The listing builds one solid part. Answer for the finished solid, in the listing's coordinates (mm). A direction names the side the tool comes from. Round coordinates to 2 decimals unless told otherwise and drop trailing zeros. Order: outer loops, then holes, each group sorted by start corner. A loop starts at its lowest first (then second) coordinate and runs counter-clockwise, first axis right, second up. Notation, with made-up numbers: (-2, -13) -> (51, -13) arc R22 ccw to (51, 25) -> close; hole circle Ø10 at (-4.5, -34.75). An arc over 180 degrees is marked (long way). Return JSON: item names as keys, results as strings. Group by question number.
(1) Which of the six approach directions +Z, -Z, +X, -X, +Y, -Y give full straight-line access (tool end or side, diameter ignored) to faces 5 (the face through (1589.699, -64, 595)), 6 (the face through (2161.199, -69, 594))?
(2) The part is cut by section A-A (z = 535.5). Determine the outline of the cut face in (x, y) (3 decimals), plus the area to 3 significant figures.
(3) The part is cut by section D-D (x = 1942.5). Determine the outline of the cut face in (y, z) (3 decimals), plus the area to 3 significant figures.
(4) Consider line 1 (Z direction, x = 1769, y = -71.5); line 2 (X direction, y = -91, z = 638); line 3 (Y direction, x = 1676.5, z = 332) (3 decimals). Determine where each line is inside the solid, lowest interval first. Write a range as [from, to].
(5) The part is cut by section C-C (y = -76.5). Determine the outline of the cut face in (x, z).
(6) Determine the mould class of faces 1 (the face through (1840.956, 4.696, 556.211)), 2 (the face through (1899, -64, 895.149)), 3 (the face through (1890, -64, 285.549)), 4 (the face through (1898, -69, 323.649)) for opening direction Z: +Z half, -Z half, draft (parallel to the pull), parting line (faces both ways), or undercut.
(7) The part is cut by section B-B (x = 1684). Determine the outline of the cut face in (y, z) (3 decimals), plus the area to 3 significant figures.
(8) This flat-tipped pin is pushed along its axis until it touches: pin 1 (2 mm diameter, centred on x = 1862, z = 490.5, fed in from -Y). Where does it stop, or does it pass through?
from build123d import *

# Parameters (mm, degrees)
SKETCH1_W           = 609.6
SKETCH1_H           = 609.6
SKETCH1_R           = 63.5
BOSS_EXTRUDE1_DEPTH = 9.525
BOSS_EXTRUDE2_DEPTH = 139.7


with BuildPart() as part:
    # Sketch1 → Boss-Extrude1 (new body)
    with BuildSketch(Plane(origin=(0, 0, 0), x_dir=(1, 0, 0), z_dir=(0, 1, 0))):
        with Locations((1894.49897269, -590.348674534)):
            Rectangle(SKETCH1_W, SKETCH1_H)
        with Locations(Location((1894.49897269, -590.348674534, 0), (0, 0, 90))):
            Circle(SKETCH1_R, mode=Mode.SUBTRACT)
    extrude(amount=BOSS_EXTRUDE1_DEPTH)

    # Sketch2 → Boss-Extrude2 (add)
    with BuildSketch(Plane.XZ):
        Polygon((1589.69897269, 323.648674534), (1589.69897269, 285.548674534), (1742.09897269, 285.548674534), (2046.89897269, 285.548674534), (2199.29897269, 285.548674534), (2199.29897269, 437.948674534), (2199.29897269, 742.748674534), (2199.29897269, 895.148674534), (2046.89897269, 895.148674534), (1742.09897269, 895.148674534), (1589.69897269, 895.148674534), (1589.69897269, 742.748674534), (1589.69897269, 437.948674534), align=None)
        Polygon((1742.09897269, 323.648674534), (1627.79897269, 323.648674534), (1627.79897269, 437.948674534), (1627.79897269, 742.748674534), (1627.79897269, 857.048674534), (1742.09897269, 857.048674534), (2046.89897269, 857.048674534), (2161.19897269, 857.048674534), (2161.19897269, 742.748674534), (2161.19897269, 437.948674534), (2161.19897269, 323.648674534), (2046.89897269, 323.648674534), align=None, mode=Mode.SUBTRACT)
    extrude(amount=BOSS_EXTRUDE2_DEPTH)


solid = part.part
Answer below:
{
 "1": {"face 5": "+Z, -Z, -X, +Y, -Y", "face 6": "-Y"},
 "2": {"outline": "(1589.699, -139.7) -> (1627.799, -139.7) -> (1627.799, 0) -> (1862.501, 0) -> (1862.501, 9.525) -> (1589.699, 9.525) -> close; (1926.497, 0) -> (2161.199, 0) -> (2161.199, -139.7) -> (2199.299, -139.7) -> (2199.299, 9.525) -> (1926.497, 9.525) -> close", "area": "15,800 mm²"},
 "3": {"outline": "(-139.7, 285.549) -> (9.525, 285.549) -> (9.525, 548.778) -> (0, 548.778) -> (0, 323.649) -> (-139.7, 323.649) -> close; (-139.7, 857.049) -> (0, 857.049) -> (0, 631.92) -> (9.525, 631.92) -> (9.525, 895.149) -> (-139.7, 895.149) -> close", "area": "15,700 mm²"},
 "4": {"line 1": "z = [285.55, 323.65], [857.05, 895.15]", "line 2": "x = [1589.7, 1627.8], [2161.2, 2199.3]", "line 3": "y = [0, 9.525]"},
 "5": {"outline": "(1589.7, 285.55) -> (2199.3, 285.55) -> (2199.3, 895.15) -> (1589.7, 895.15) -> close; hole (1627.8, 323.65) -> (2161.2, 323.65) -> (2161.2, 857.05) -> (1627.8, 857.05) -> close"},
 "6": {"face 1": "undercut", "face 2": "+Z half", "face 3": "-Z half", "face 4": "undercut"},
 "7": {"outline": "(-139.7, 285.549) -> (9.525, 285.549) -> (9.525, 895.149) -> (-139.7, 895.149) -> (-139.7, 857.049) -> (0, 857.049) -> (0, 323.649) -> (-139.7, 323.649) -> close", "area": "16,500 mm²"},
 "8": {"pin 1": "stops at y = 0"}
}
